The drawing under review shows one solid part. Ordinate dimensions are in mm from its lowest x, y, z. Give positions to 0.01 mm unless a question says otherwise; leave off trailing zeros. Order: outer loops, then holes, each group sorted by start corner. A loop starts at its lowest first (then second) coordinate and runs counter-clockwise, first axis right, second up. Notation, with made-up numbers: (48, 55.25) - (72, 55.25) arc R36 ccw to (72, 89.25) - close; hole circle Ø11 at (-24.75, -30). An arc over 180 degrees is marked (long way). Write item = value, one per line. Start each with the question number.
1. We need section B-B, the plane y = 2.1. Give the boundary of the cut face in (x, z) (1 decimal).
2. Wall thickness on probe 1 along Z at (x, y) = (12.7, 0.7); probe 2 along Z at (x, y) = (9.75, 2.25) (1 decimal); probe 3 along X at (y, z) = (0.6, 39): over which ranges is each line inside the solid? List them lowest first.
3. We need section A-A, the plane z = 12.7. Give the boundary of the cut face in (x, y) (1 decimal).
4. We need section D-D, the plane z = 36. Give the boundary of the cut face in (x, y) (1 decimal).
5. We need section C-C, the plane x = 12.7. Give the boundary of the cut face in (y, z) (1 decimal), and give its area (3 significant figures).
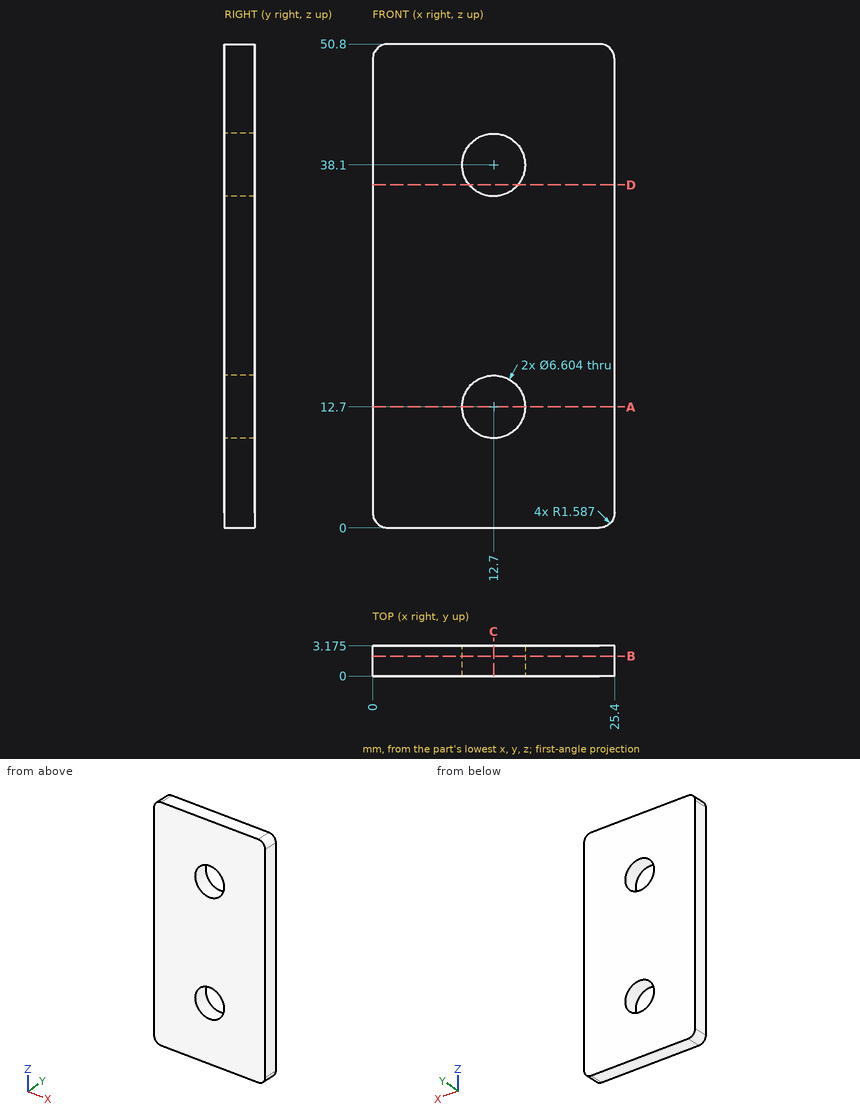
Model answer:
q1.outline = (0, 1.6) arc R1.6 ccw to (1.6, 0) - (23.8, 0) arc R1.6 ccw to (25.4, 1.6) - (25.4, 49.2) arc R1.6 ccw to (23.8, 50.8) - (1.6, 50.8) arc R1.6 ccw to (0, 49.2) - close; hole circle Ø6.6 at (12.7, 12.7); hole circle Ø6.6 at (12.7, 38.1)
q2.probe_1 = 0 to 9.4, 16 to 34.8, 41.4 to 50.8
q2.probe_2 = 0 to 11.2, 14.2 to 36.6, 39.6 to 50.8
q2.probe_3 = 0 to 9.52, 15.88 to 25.4
q3.outline = (0, 0) - (9.4, 0) - (9.4, 3.2) - (0, 3.2) - close; (16, 0) - (25.4, 0) - (25.4, 3.2) - (16, 3.2) - close
q4.outline = (0, 0) - (10.2, 0) - (10.2, 3.2) - (0, 3.2) - close; (15.2, 0) - (25.4, 0) - (25.4, 3.2) - (15.2, 3.2) - close
q5.outline = (0, 0) - (3.2, 0) - (3.2, 9.4) - (0, 9.4) - close; (0, 16) - (3.2, 16) - (3.2, 34.8) - (0, 34.8) - close; (0, 41.4) - (3.2, 41.4) - (3.2, 50.8) - (0, 50.8) - close
q5.area = 119 mm2
